The model under review builds one solid part; all positions refer to its coordinate system, in mm. A direction names the side the tool comes from. Round coordinates to 2 decimals unless told otherwise and drop trailing zeros. Order: outer loops, then holes, each group sorted by start corner. A loop starts at its lowest first (then second) coordinate and runs counter-clockwise, first axis right, second up. Notation, with made-up numbers: M 32.25,38.5 L 88.25,38.5 A27 cw 88.25,61.5 Z; hole C -27.75,-15 d2. An arc over 180 degrees is marked long. Answer as a JSON object with one key per item and string values. Group by question number.
1. Add section C-C on z = 9. State the section outline as (x, y) points, and give its area (3 significant figures).
2. Machinability: for faces 1 (the face through (4, 0, 21)), 2 (the face through (-4.95, 0.03, 14.71)), 3 (the face through (0, -5, 20)), 4 (the face through (-0.54, -2.44, -0.39)), 5 (the face through (1, 0, 31)), which of the approach directions +Z, -Z, +X, -X, +Y, -Y give a long, thin tool a straight path to every point of the face, cutting with its end or side? Answer none if there is none.
3. Add section D-D on x = -4.5. State the section outline as (y, z) points, and give its area (3 significant figures).
4. Add section B-B on y = -3.5. State the section outline as (x, z) points, and give its area (3 significant figures).
5. Clearance check with flat-ended pins moving along their axes: P1, Ø2.5, axis at x = -0.5, y = 0.5, coming from the -Z side; P2, Ø3, axis at x = 4, y = -1.5, coming from the +Z side; P3, Ø1.2, axis at y = 0, z = -1, coming from the +X side. State where each tip first meets the part, or that it passes through.
6. Add section A-A on x = 3. State the section outline as (y, z) points.
7. Mouldability with a two-part tool opening along Y and no side actions: class faces 6 (the face through (0, 5, 20)), 7 (the face through (-4.5, 0, 18.41)), 8 (the face through (6, 0, 20)) as released by +Y, released by -Y, zero draft, split by the parting line, or undercut.
8. To check wall thickness, follow probe 1 along Y at (x, z) = (4.5, 22.7); probe 2 along Y at (x, z) = (0, 14.9); probe 3 along Z at (x, y) = (5.75, -2). State the ranges of each line that lie inside material, in increasing order. Write a range as [from, to].
```python
from build123d import *

# Parameters (mm, degrees)
SKETCH_1_W          = 0.3
SKETCH_1_H          = 1.5
SKETCH_1_R          = 2.5
SKETCH_1_R_2        = 1.5
EXTRUDE_1_DEPTH     = 15.2
SKETCH_1_4_W        = 0.3
SKETCH_1_4_H        = 1.5
EXTRUDE_2_DEPTH     = 2
CUT_EXTRUDE_2_DEPTH = 19.763794925
FILLET_1_R          = 0.4
SKETCH_1_5_R        = 2.5
SKETCH_1_5_R_2      = 1.5
EXTRUDE_3_DEPTH     = 1.2
CUT_EXTRUDE_START   = -1.2
SKETCH_1_7_R        = 1.5
CUT_EXTRUDE_1_DEPTH = 0.6
FILLET_2_R          = 0.4
SKETCH_3_R          = 2
EXTRUDE_4_DEPTH     = 0.5
SKETCH_3_3_R        = 0.5
EXTRUDE_5_DEPTH     = 3
SKETCH_4_R          = 0.7
SKETCH_4_R_2        = 0.5
CUT_EXTRUDE_3_DEPTH = 1
EXTRUDE_START       = 0.01
SKETCH_5_W          = 12
SKETCH_5_H          = 10
EXTRUDE_6_DEPTH     = 9
SKETCH_6_R          = 2
EXTRUDE_7_DEPTH     = 0.2
SKETCH_6_4_R        = 1.5
EXTRUDE_8_DEPTH     = 4
EXTRUDE_START_2     = 4
EXTRUDE_9_DEPTH     = 6
SKETCH_7_R          = 0.5
CUT_EXTRUDE_5_DEPTH = 5.8


with BuildPart() as part:
    # 草图1 → 凸台-拉伸1 (new body)
    # profile 1 of 5: a face of its own
    with BuildSketch(Plane.XY):
        with BuildLine():
            ThreePointArc((-6, 0), (-5.286764074, -2.837274331), (-3.31662479, -5))
            Line((-3.31662479, -5), (3.31662479, -5))
            ThreePointArc((3.31662479, -5), (5.286764074, -2.837274331), (6, 0))
            ThreePointArc((6, 0), (5.286764074, 2.837274331), (3.31662479, 5))
            Line((3.31662479, 5), (-3.31662479, 5))
            ThreePointArc((-3.31662479, 5), (-5.286764074, 2.837274331), (-6, 0))
        make_face()
        with Locations((-3.65, 0)):
            Rectangle(SKETCH_1_W, SKETCH_1_H, mode=Mode.SUBTRACT)
        Circle(SKETCH_1_R, mode=Mode.SUBTRACT)
        with Locations((3.65, 0)):
            Rectangle(SKETCH_1_W, SKETCH_1_H, mode=Mode.SUBTRACT)
    # profile 2 of 5: a face of its own
    with BuildSketch(Plane.XY):
        Circle(SKETCH_1_R)
        Circle(SKETCH_1_R_2, mode=Mode.SUBTRACT)
    # profile 3 of 5: a face of its own
    with BuildSketch(Plane.XY):
        Circle(SKETCH_1_R_2)
    # profile 4 of 5: a face of its own
    with BuildSketch(Plane.XY):
        with Locations((3.65, 0)):
            Rectangle(SKETCH_1_W, SKETCH_1_H)
    # profile 5 of 5: a face of its own
    with BuildSketch(Plane.XY):
        with Locations((-3.65, 0)):
            Rectangle(SKETCH_1_W, SKETCH_1_H)
    extrude(amount=EXTRUDE_1_DEPTH)

    # 草图1<4> → 凸台-拉伸2 (add)
    with BuildSketch(Plane.XY):
        with Locations((3.65, 0)):
            Rectangle(SKETCH_1_4_W, SKETCH_1_4_H)
        with Locations((-3.65, 0)):
            Rectangle(SKETCH_1_4_W, SKETCH_1_4_H)
    extrude(amount=-EXTRUDE_2_DEPTH)

    # 草图2 → 切除-拉伸2 (cut, through all)
    with BuildSketch(Plane(origin=(3.8, 0, 0), x_dir=(0, 0, -1), z_dir=(1, 0, 0))):
        with BuildLine():
            Line((0.95, 0.45), (1.05, 0.45))
            ThreePointArc((1.05, 0.45), (1.5, 0), (1.05, -0.45))
            Line((1.05, -0.45), (0.95, -0.45))
            ThreePointArc((0.95, -0.45), (0.5, 0), (0.95, 0.45))
        make_face()
    extrude(amount=-CUT_EXTRUDE_2_DEPTH, mode=Mode.SUBTRACT)

    # 圆角1
    fillet_1_edges = [part.edges().sort_by_distance(p)[0] for p in [
        (3.65, -0.75, -2),
        (3.65, 0.75, -2),
        (-3.65, -0.75, -2),
        (-3.65, 0.75, -2),
    ]]
    fillet(fillet_1_edges, radius=FILLET_1_R)

    # 草图1<5> → 凸台-拉伸3 (add)
    # profile 1 of 2: a face of its own
    with BuildSketch(Plane.XY):
        Circle(SKETCH_1_5_R)
        Circle(SKETCH_1_5_R_2, mode=Mode.SUBTRACT)
    # profile 2 of 2: a face of its own
    with BuildSketch(Plane.XY):
        Circle(SKETCH_1_5_R_2)
    extrude(amount=-EXTRUDE_3_DEPTH)

    # 草图1<7> → 切除-拉伸1 (cut)
    with BuildSketch(Plane.XY.offset(CUT_EXTRUDE_START)):
        Circle(SKETCH_1_7_R)
    extrude(amount=CUT_EXTRUDE_1_DEPTH, mode=Mode.SUBTRACT)

    # 圆角2
    fillet_2_edges = [part.edges().sort_by_distance(p)[0] for p in [
        (-2.5, 0, -1.2),
    ]]
    fillet(fillet_2_edges, radius=FILLET_2_R)

    # 草图3 → 凸台-拉伸4 (add)
    with BuildSketch(Plane.XY.offset(15.2)):
        Circle(SKETCH_3_R)
    extrude(amount=EXTRUDE_4_DEPTH)

    # 草图3<3> → 凸台-拉伸5 (add)
    with BuildSketch(Plane.XY.offset(15.2)):
        Circle(SKETCH_3_3_R)
    extrude(amount=EXTRUDE_5_DEPTH)

    # 草图4 → 切除-拉伸3 (cut)
    with BuildSketch(Plane.XY.offset(15.2)):
        with Locations((-4.25, 0)):
            Circle(SKETCH_4_R)
        with Locations((4.25, 0)):
            Circle(SKETCH_4_R)
        with Locations((0, 3.5)):
            Circle(SKETCH_4_R_2)
    extrude(amount=-CUT_EXTRUDE_3_DEPTH, mode=Mode.SUBTRACT)

    # 草图5 → 凸台-拉伸6 (add)
    with BuildSketch(Plane.XY.offset(15.2).offset(EXTRUDE_START)):
        Rectangle(SKETCH_5_W, SKETCH_5_H)
    extrude(amount=EXTRUDE_6_DEPTH)

    # 草图6 → 凸台-拉伸7 (add)
    with BuildSketch(Plane.XY.offset(24.21)):
        Circle(SKETCH_6_R)
    extrude(amount=EXTRUDE_7_DEPTH)

    # 草图6<4> → 凸台-拉伸8 (add)
    with BuildSketch(Plane.XY.offset(24.21)):
        Circle(SKETCH_6_4_R)
    extrude(amount=EXTRUDE_8_DEPTH)

    # 草图6<5> → 凸台-拉伸9 (add)
    with BuildSketch(Plane.XY.offset(24.21).offset(EXTRUDE_START_2)):
        with BuildLine():
            Line((1, -1.118033989), (1, 1.118033989))
            ThreePointArc((1, 1.118033989), (-1.5, 0), (1, -1.118033989))
        make_face()
    extrude(amount=EXTRUDE_9_DEPTH)

    # 草图7 → 切除-拉伸5 (cut)
    with BuildSketch(Plane.XY.offset(24.21)):
        with Locations((-4.5, 0)):
            Circle(SKETCH_7_R)
        with Locations((4.5, 0)):
            Circle(SKETCH_7_R)
    extrude(amount=-CUT_EXTRUDE_5_DEPTH, mode=Mode.SUBTRACT)


solid = part.part
```
Recorded:
{
 "1": {"outline": "M -3.32,-5 L 3.32,-5 A6 ccw 3.32,5 L -3.32,5 A6 ccw Z", "area": "104 mm²"},
 "2": {"face 1": "+Z", "face 2": "none", "face 3": "+Z, -Z, +X, -X, -Y", "face 4": "-Z", "face 5": "+Z, +X, +Y, -Y"},
 "3": {"outline": "M -5,15.21 L 5,15.21 L 5,24.21 L 0.5,24.21 L 0.5,18.41 L -0.5,18.41 L -0.5,24.21 L -5,24.21 Z; M -3.97,0 L 3.97,0 L 3.97,15.2 L 0.65,15.2 L 0.65,14.2 L -0.65,14.2 L -0.65,15.2 L -3.97,15.2 Z", "area": "204 mm²"},
 "4": {"outline": "M -6,15.21 L 6,15.21 L 6,24.21 L -6,24.21 Z; M -4.87,0 L 4.87,0 L 4.87,15.2 L -4.87,15.2 Z", "area": "256 mm²"},
 "5": {"P1": "stops at z = -1.2", "P2": "stops at z = 24.21", "P3": "stops at x = 3.8"},
 "6": {"outline": "M -5,0 L 5,0 L 5,15.2 L -5,15.2 Z; M -5,15.21 L 5,15.21 L 5,24.21 L -5,24.21 Z"},
 "7": {"face 6": "released by +Y", "face 7": "undercut", "face 8": "zero draft"},
 "8": {"probe 1": "y = [-5, -0.5], [0.5, 5]", "probe 2": "y = [-5, 3], [4, 5]", "probe 3": "z = [15.21, 24.21]"}
}
